Geometry check sheet. Reference: the model listing, model coordinates, mm. A direction names the side the tool comes from. Give positions to 0.01 mm unless a question says otherwise; leave off trailing zeros. Write each loop counter-clockwise with the first axis right and the second up, starting at its lowest first coordinate (ties: lowest second). Pieces come first, ordered by that corner, then holes.
(1) Cross-section at A-A (y = -1). Record the boundary of the cut face in (x, z).
(2) Thickness scan on line 1 along X through (y, z) = (-1.85, 0); line 2 along Z through (x, y) = (0, -1.5); line 3 along X through (y, z) = (-2.8, 0.25). Record the ranges inside material, lowest first.
(3) Mould release check, pull along X, two halves, no side actions. Record for faces 1 (the flat face through (4, -0.8, 0)), 2 (the cylindrical face through (-2.14, -0.39, -2.1)), 3 (the cylindrical face through (-1.115, -2.226, -1.216)), 4 (the conical face through (3.454, -3.629, 1.565)): +X half, -X half, draft (parallel to the pull), parting line (faces both ways), or undercut.
(4) Tool access check on faces 5 (the cylindrical face through (4.736, -1.54, 1.602)), 6 (the cylindrical face through (2.14, -0.39, 2.1)). Record the directions out of +Z, -Z, +X, -X, +Y, -Y that give a thin tool (end or side, any length) a straight path to the whole face; none if there is none.
(5) Depth check by flat-ended pin: P1, Ø1.5, axis at x = 0.5, z = 0.5, coming from the +Y side; P2, Ø2, axis at y = -0.5, z = 1, coming from the -X side. Enter the tip coordinate at first touch or a pass-through.
```python
from build123d import *

# Parameters (mm, degrees)
EXTRUDE_1_DEPTH     = 3
CUT_EXTRUDE_1_DEPTH = 0.8
CUT_EXTRUDE_2_DEPTH = 4.7


with BuildPart() as part:
    # Эскиз1 → Бобышка-Вытянуть1 (new body, symmetric)
    with BuildSketch(Plane.XY):
        Polygon((3, 0), (-3, 0), (-3, -0.8), (-5, -0.8), (-5, -4.5), (5, -4.5), (5, -0.8), (3, -0.8), align=None)
    extrude(amount=EXTRUDE_1_DEPTH, both=True)

    # Эскиз3 → Отверстие обработанное метчиком M41 (revolve, cut)
    with BuildSketch(Plane(origin=(0, 0, 0), x_dir=(0, 0, 1), z_dir=(1, 0, 0))):
        Polygon((0, 0), (0, 4.5), (2.15, 4.5), (1.65, 4), (1.65, 0.5), (2.15, 0), align=None)
    revolve(axis=Axis((0, 6.35, 0), (0, -1, 0)), mode=Mode.SUBTRACT)

    # Эскиз4 → Вырез-Вытянуть1 (cut)
    with BuildSketch(Plane(origin=(0, 0, 0), x_dir=(1, 0, 0), z_dir=(0, 1, 0))):
        with BuildLine():
            Line((-3, 3), (-3, 0))
            ThreePointArc((-3, 0), (-2.121320344, 2.121320344), (0, 3))
            Line((0, 3), (-3, 3))
        make_face()
        with BuildLine():
            Line((0, -3), (3, -3))
            Line((3, -3), (3, 0))
            ThreePointArc((3, 0), (2.121320344, -2.121320344), (0, -3))
        make_face()
    extrude(amount=-CUT_EXTRUDE_1_DEPTH, mode=Mode.SUBTRACT)

    # Эскиз5 → Вырез-Вытянуть2 (cut, through all)
    with BuildSketch(Plane(origin=(0, -0.8, 0), x_dir=(1, 0, 0), z_dir=(0, 1, 0))):
        with BuildLine():
            Line((-5, 0), (-5, 3))
            Line((-5, 3), (-4, 3))
            ThreePointArc((-4, 3), (-4.74341649, 1.58113883), (-5, 0))
        make_face()
        with BuildLine():
            Line((5, 0), (5, -3))
            Line((5, -3), (4, -3))
            ThreePointArc((4, -3), (4.74341649, -1.58113883), (5, 0))
        make_face()
    extrude(amount=-CUT_EXTRUDE_2_DEPTH, mode=Mode.SUBTRACT)

    # Вырез-По траектории1: sweep along a path in Эскиз7
    with BuildLine(Plane.XZ.offset(4.5)) as sweep_1_path:
        Line((0, 5), (-5, 5))
        Line((-5, 5), (-5, 0))
        ThreePointArc((-5, 0), (-3.535533906, -3.535533906), (0, -5))
        Line((0, -5), (5, -5))
        Line((5, -5), (5, 0))
        ThreePointArc((5, 0), (3.535533906, 3.535533906), (0, 5))
    # Эскиз6 → Вырез-По траектории1 (sweep, cut)
    with BuildSketch(Plane.XY.offset(3)):
        Polygon((-5, -2.3), (-5, -4.5), (-3, -4.5), align=None)
    sweep(path=sweep_1_path.line, transition=Transition.RIGHT, mode=Mode.SUBTRACT)


solid = part.part
```
Reply:
1. outline: (-5, 0) arc R5 ccw to (-4, -3) - (5, -3) - (5, 0) arc R5 ccw to (4, 3) - (-5, 3) - close; hole circle Ø3.3 at (0, 0)
2. line 1: x = -5 to -1.65, 1.65 to 5
2. line 2: z = -3 to -1.65, 1.65 to 3
2. line 3: x = -4.55 to -1.63, 1.63 to 4.54
3. face 1: draft
3. face 2: -X half
3. face 3: undercut
3. face 4: +X half
4. face 5: +Z, +X, +Y, -Y
4. face 6: +Z, +X, +Y
5. P1: passes through
5. P2: stops at x = -5
